```python
from build123d import *

# Parameters (mm, degrees)
CYLINDER531_R     = 1.5
CYLINDER531_DEPTH = 100
CYLINDER530_R     = 1.5
CYLINDER530_DEPTH = 100
CYLINDER364_R     = 1.5
CYLINDER364_DEPTH = 50
CYLINDER363_R     = 3
CYLINDER363_DEPTH = 4
BOX135_W          = 200
BOX135_H          = 100
BOX135_DEPTH      = 32
CYLINDER328_R     = 1.5
CYLINDER328_DEPTH = 50
CYLINDER330_R     = 1.5
CYLINDER330_DEPTH = 50
CYLINDER331_R     = 1.5
CYLINDER331_DEPTH = 50
CYLINDER329_R     = 1.5
CYLINDER329_DEPTH = 50
CYLINDER334_R     = 3
CYLINDER334_DEPTH = 4
CYLINDER327_R     = 3
CYLINDER327_DEPTH = 4
CYLINDER292_R     = 1.5
CYLINDER292_DEPTH = 100
CYLINDER291_R     = 1.5
CYLINDER291_DEPTH = 100
CYLINDER316_R     = 3
CYLINDER316_DEPTH = 4
CYLINDER315_R     = 3
CYLINDER315_DEPTH = 4
CYLINDER313_R     = 1.5
CYLINDER313_DEPTH = 50
CYLINDER314_R     = 1.5
CYLINDER314_DEPTH = 50
CYLINDER311_R     = 3
CYLINDER311_DEPTH = 4
CYLINDER312_R     = 3
CYLINDER312_DEPTH = 4
TUBE_R            = 59
TUBE_R_2          = 40
TUBE_DEPTH        = 10


with BuildPart() as obj1:
    # Cylinder531 → Cylinder531 (new body)
    with BuildSketch(Plane(origin=(39, -21, 0), x_dir=(1, 0, 0), z_dir=(0, 0, 1))):
        Circle(CYLINDER531_R)
    extrude(amount=CYLINDER531_DEPTH)


with BuildPart() as compound308:
    # Cylinder530 → Cylinder530 (new body)
    with BuildSketch(Plane(origin=(-39, -21, 0), x_dir=(1, 0, 0), z_dir=(0, 0, 1))):
        Circle(CYLINDER530_R)
    extrude(amount=CYLINDER530_DEPTH)

    # Compound308: union obj1
    add(obj1.part)


with BuildPart() as obj2:
    # Cylinder364 → Cylinder364 (new body)
    with BuildSketch(Plane(origin=(0, 50, 0), x_dir=(1, 0, 0), z_dir=(0, 0, 1))):
        Circle(CYLINDER364_R)
    extrude(amount=CYLINDER364_DEPTH)


with BuildPart() as obj3:
    # Cylinder363 → Cylinder363 (new body)
    with BuildSketch(Plane(origin=(0, 50, -1), x_dir=(1, 0, 0), z_dir=(0, 0, 1))):
        Circle(CYLINDER363_R)
    extrude(amount=CYLINDER363_DEPTH)


with BuildPart() as krychle135:
    # Box135 → Box135 (new body)
    with BuildSketch(Plane(origin=(-100, -124, 0), x_dir=(1, 0, 0), z_dir=(0, 0, 1))):
        with Locations((100, 50)):
            Rectangle(BOX135_W, BOX135_H)
    extrude(amount=BOX135_DEPTH)


with BuildPart() as obj4:
    # Cylinder328 → Cylinder328 (new body)
    with BuildSketch(Plane(origin=(-51, 6, 0), x_dir=(1, 0, 0), z_dir=(0, 0, 1))):
        Circle(CYLINDER328_R)
    extrude(amount=CYLINDER328_DEPTH)


with BuildPart() as obj5:
    # Cylinder330 → Cylinder330 (new body)
    with BuildSketch(Plane(origin=(-24, 18, 0), x_dir=(1, 0, 0), z_dir=(0, 0, 1))):
        Circle(CYLINDER330_R)
    extrude(amount=CYLINDER330_DEPTH)


with BuildPart() as obj6:
    # Cylinder331 → Cylinder331 (new body)
    with BuildSketch(Plane(origin=(24, 18, 0), x_dir=(1, 0, 0), z_dir=(0, 0, 1))):
        Circle(CYLINDER331_R)
    extrude(amount=CYLINDER331_DEPTH)


with BuildPart() as compound297:
    # Cylinder329 → Cylinder329 (new body)
    with BuildSketch(Plane(origin=(51, 6, 0), x_dir=(1, 0, 0), z_dir=(0, 0, 1))):
        Circle(CYLINDER329_R)
    extrude(amount=CYLINDER329_DEPTH)

    # Compound297: union obj4, obj5, obj6
    add(obj4.part)
    add(obj5.part)
    add(obj6.part)


with BuildPart() as obj7:
    # Cylinder334 → Cylinder334 (new body)
    with BuildSketch(Plane(origin=(24, 18, 0), x_dir=(1, 0, 0), z_dir=(0, 0, 1))):
        Circle(CYLINDER334_R)
    extrude(amount=CYLINDER334_DEPTH)


with BuildPart() as compound298:
    # Cylinder327 → Cylinder327 (new body)
    with BuildSketch(Plane(origin=(-24, 18, 0), x_dir=(1, 0, 0), z_dir=(0, 0, 1))):
        Circle(CYLINDER327_R)
    extrude(amount=CYLINDER327_DEPTH)

    # Compound298: union obj7
    add(obj7.part)


with BuildPart() as compound298_1:
    # Compound298 placement: moved
    add(compound298.part.moved(Location((0, 0, 7))))


with BuildPart() as obj8:
    # Cylinder292 → Cylinder292 (new body)
    with BuildSketch(Plane(origin=(51, -12, 0), x_dir=(1, 0, 0), z_dir=(0, 0, 1))):
        Circle(CYLINDER292_R)
    extrude(amount=CYLINDER292_DEPTH)


with BuildPart() as compound292:
    # Cylinder291 → Cylinder291 (new body)
    with BuildSketch(Plane(origin=(-51, -12, 0), x_dir=(1, 0, 0), z_dir=(0, 0, 1))):
        Circle(CYLINDER291_R)
    extrude(amount=CYLINDER291_DEPTH)

    # Compound292: union obj8
    add(obj8.part)


with BuildPart() as obj9:
    # Cylinder316 → Cylinder316 (new body)
    with BuildSketch(Plane(origin=(51, -16, 0), x_dir=(1, 0, 0), z_dir=(0, 0, 1))):
        Circle(CYLINDER316_R)
    extrude(amount=CYLINDER316_DEPTH)


with BuildPart() as compound293:
    # Cylinder315 → Cylinder315 (new body)
    with BuildSketch(Plane(origin=(-51, -16, 0), x_dir=(1, 0, 0), z_dir=(0, 0, 1))):
        Circle(CYLINDER315_R)
    extrude(amount=CYLINDER315_DEPTH)

    # Compound293: union obj9
    add(obj9.part)


with BuildPart() as compound293_1:
    # Compound293 placement: moved
    add(compound293.part.moved(Location((0, 0, 25))))


with BuildPart() as obj10:
    # Cylinder313 → Cylinder313 (new body)
    with BuildSketch(Plane(origin=(34, 36, 0), x_dir=(1, 0, 0), z_dir=(0, 0, 1))):
        Circle(CYLINDER313_R)
    extrude(amount=CYLINDER313_DEPTH)


with BuildPart() as compound291:
    # Cylinder314 → Cylinder314 (new body)
    with BuildSketch(Plane(origin=(-34, 36, 0), x_dir=(1, 0, 0), z_dir=(0, 0, 1))):
        Circle(CYLINDER314_R)
    extrude(amount=CYLINDER314_DEPTH)

    # Compound291: union obj10
    add(obj10.part)


with BuildPart() as obj11:
    # Cylinder311 → Cylinder311 (new body)
    with BuildSketch(Plane(origin=(-34, 36, -1), x_dir=(1, 0, 0), z_dir=(0, 0, 1))):
        Circle(CYLINDER311_R)
    extrude(amount=CYLINDER311_DEPTH)


with BuildPart() as compound290:
    # Cylinder312 → Cylinder312 (new body)
    with BuildSketch(Plane(origin=(34, 36, -1), x_dir=(1, 0, 0), z_dir=(0, 0, 1))):
        Circle(CYLINDER312_R)
    extrude(amount=CYLINDER312_DEPTH)

    # Compound290: union obj11
    add(obj11.part)


with BuildPart() as cut169:
    # Tube → Tube (new body)
    with BuildSketch(Plane.XY):
        Circle(TUBE_R)
        Circle(TUBE_R_2, mode=Mode.SUBTRACT)
    extrude(amount=TUBE_DEPTH)

    # Cut136: cut Compound290
    add(compound290.part, mode=Mode.SUBTRACT)

    # Cut137: cut Compound291
    add(compound291.part, mode=Mode.SUBTRACT)

    # Cut138: cut Compound293
    add(compound293_1.part, mode=Mode.SUBTRACT)

    # Cut139: cut Compound292
    add(compound292.part, mode=Mode.SUBTRACT)

    # Cut142: cut Compound298
    add(compound298_1.part, mode=Mode.SUBTRACT)

    # Cut143: cut Compound297
    add(compound297.part, mode=Mode.SUBTRACT)

    # Cut144: cut Krychle135
    add(krychle135.part, mode=Mode.SUBTRACT)

    # Cut153: cut obj3
    add(obj3.part, mode=Mode.SUBTRACT)

    # Cut154: cut obj2
    add(obj2.part, mode=Mode.SUBTRACT)

    # Cut169: cut Compound308
    add(compound308.part, mode=Mode.SUBTRACT)


solid = cut169.part
```
Input: part model. Units: mm. Frame: model coordinates. A direction names the side the tool comes from. Round coordinates to 2 decimals unless told otherwise and drop trailing zeros. Order: outer loops, then holes, each group sorted by start corner. A loop starts at its lowest first (then second) coordinate and runs counter-clockwise, first axis right, second up. Notation, with made-up numbers: (-40, -35) - (18, -35) arc R18 ccw to (18, -25) - close; hole circle Ø6 at (-40, 4). An arc over 180 degrees is marked (long way). Answer in a Markdown table with one row per item.
Item 1: Mould query, pull axis X, two halves, no side actions, for faces 1 (the flat face through (-1, 46, 0)), 2 (the cylindrical face through (1.24, 39.98, 4.93)), 3 (the cylindrical face through (1.643, 58.977, 4.93)), 4 (the flat face through (-32.7, 34.7, 3)). Classes: released by +X, released by -X, zero draft, split by the parting line, or undercut.
Model answer:
| item | result |
|---|---|
| face 1 | zero draft |
| face 2 | undercut |
| face 3 | split by the parting line |
| face 4 | undercut |
Item 2: Pin query (flat end, axial travel): pin 1 (2.5 mm diameter, centred on x = 39, y = -21, fed in from +Z); pin 2 (5 mm diameter, centred on x = -9.5, z = 2.5, fed in from +Y); pin 3 (5 mm diameter, centred on x = 20.5, z = 6.5, fed in from +Y); pin 4 (4 mm diameter, centred on y = 13.5, z = 5, fed in from -X). Return the tip coordinate at first contact, or that it passes through.
Model answer:
| item | result |
|---|---|
| pin 1 | passes through |
| pin 2 | stops at y = 58.58 |
| pin 3 | stops at y = 56.19 |
| pin 4 | stops at x = -57.87 |
Item 3: Section query C-C (x = 51). Return the cut outline in (y, z).
Model answer:
| item | result |
|---|---|
| outline | (-24, 0) - (-13.5, 0) - (-13.5, 10) - (-24, 10) - close; (-10.5, 0) - (4.5, 0) - (4.5, 10) - (-10.5, 10) - close; (7.5, 0) - (29.66, 0) - (29.66, 10) - (7.5, 10) - close |
Item 4: Section query A-A (y = 0). Return the cut outline in (x, z), then the cut area to 3 significant figures.
Model answer:
| item | result |
|---|---|
| outline | (-59, 0) - (-40, 0) - (-40, 10) - (-59, 10) - close; (40, 0) - (59, 0) - (59, 10) - (40, 10) - close |
| area | 380 mm² |
Item 5: Line query: line 1 (Y direction, x = 0, z = 4.25); line 2 (X direction, y = 36, z = 4.5); line 3 (X direction, y = 6, z = 7.75). Output: solid intervals per line, ascending.
Model answer:
| item | result |
|---|---|
| line 1 | y = 40 to 48.5, 51.5 to 59 |
| line 2 | x = -46.74 to -35.5, -32.5 to -17.44, 17.44 to 32.5, 35.5 to 46.74 |
| line 3 | x = -58.69 to -52.5, -49.5 to -39.55, 39.55 to 49.5, 52.5 to 58.69 |
Item 6: Section query D-D (y = -21). Return the cut outline in (x, z), then the cut area to 3 significant figures.
Model answer:
| item | result |
|---|---|
| outline | (-55.14, 0) - (-40.5, 0) - (-40.5, 10) - (-55.14, 10) - close; (-37.5, 0) - (-34.04, 0) - (-34.04, 10) - (-37.5, 10) - close; (34.04, 0) - (37.5, 0) - (37.5, 10) - (34.04, 10) - close; (40.5, 0) - (55.14, 0) - (55.14, 10) - (40.5, 10) - close |
| area | 362 mm² |
Item 7: Section query B-B (z = 5.5). Give the number of separate pieces and of enclosed holes in the cut face, then the cut area to 3 significant figures.
Model answer:
| item | result |
|---|---|
| separate pieces | 1 |
| enclosed holes | 9 |
| area | 3,850 mm² |
Item 8: Reachability of faces 5 (the flat face through (-1, 46, 10)), 6 (the cylindrical face through (-36.21, 38.03, 1.48)) from +Z, -Z, +X, -X, +Y, -Y: full face, straight path, thin tool, end or side. Return the list, or none.
Model answer:
| item | result |
|---|---|
| face 5 | +Z, +X, -X, +Y, -Y |
| face 6 | -Z |
